Geometry: final body of the model. Coordinates: model frame, mm. Round coordinates to 2 decimals unless told otherwise and drop trailing zeros. Loops run counter-clockwise (first coordinate to the right, second up) from the corner with the lowest first, then second, coordinate; pieces in that order, holes last. Notation, with made-up numbers: M 65.5,-24 L 115.5,-24 A13 cw 115.5,-14 Z; hole C -20.75,21 d2. An arc over 180 degrees is marked long. Return JSON: item names as keys, results as strings.
from build123d import *

# Parameters (mm, degrees)
F0_W     = 158.75
F0_H     = 209.55
F1_DEPTH = 45
F3_DEPTH = 304.8
F4_R     = 5.08


with BuildPart() as f1:
    # F0 (on Top) → F1 (new body)
    with BuildSketch(Plane.XY):
        Rectangle(F0_W, F0_H)
    extrude(amount=F1_DEPTH)

    # F2 (on face) → F3 (join)
    with BuildSketch(Plane.XY.offset(45)):
        with BuildLine():
            Line((0, 69.9373111129), (0, 74.4373111129))
            ThreePointArc((0, 74.4373111129), (-4.5, 69.9373111129), (0, 65.4373111129))
            Line((0, 65.4373111129), (0, 69.9373111129))
        make_face()
        with BuildLine():
            ThreePointArc((4.5, 69.9373111129), (3.1819805153, 73.1192916282), (0, 74.4373111129))
            Line((0, 74.4373111129), (0, 69.9373111129))
            Line((0, 69.9373111129), (0, 65.4373111129))
            ThreePointArc((0, 65.4373111129), (3.1819805153, 66.7553305975), (4.5, 69.9373111129))
        make_face()
    extrude(amount=F3_DEPTH)

    # F4
    f4_edges = [f1.edges().sort_by_distance(p)[0] for p in [
        (79.375, 0, 45),
        (0, -104.775, 45),
        (-79.375, 0, 45),
        (0, 104.775, 45),
    ]]
    fillet(f4_edges, radius=F4_R)


solid = f1.part
Q1. Material intervals for L1, parallel to Z at x = -32, y = -93; L2, parallel to X at y = 67.5, z = 72; L3, parallel to Y at x = 60, z = 44, sorted ascending.
Determined:
{"L1": "z = 0 to 45", "L2": "x = -3.78 to 3.78", "L3": "y = -102.72 to 102.72"}
Q2. Section query B-B (z = 100). Output: boundary loops of the cut face in (x, y), plus the area to 3 significant figures.
Determined:
{"outline": "C 0,69.94 d9", "area": "63.6 mm^2"}
Q3. Pin query (flat end, axial travel): pin 1 (5 mm diameter, centred on y = 10, z = 44.5, fed in from +X). Return the tip coordinate at first contact, or that it passes through.
Determined:
{"pin 1": "stops at x = 78.93"}
Q4. Section query C-C (y = -22). Output: boundary loops of the cut face in (x, z) (3 decimals), plus the area to 3 significant figures.
Determined:
{"outline": "M -79.375,0 L 79.375,0 L 79.375,39.92 A5.08 ccw 74.295,45 L -74.295,45 A5.08 ccw -79.375,39.92 Z", "area": "7,130 mm^2"}
Q5. Section query A-A (x = -50). Output: boundary loops of the cut face in (y, z) (3 decimals).
Determined:
{"outline": "M -104.775,0 L 104.775,0 L 104.775,39.92 A5.08 ccw 99.695,45 L -99.695,45 A5.08 ccw -104.775,39.92 Z"}
